```python
from build123d import *

# Parameters (mm, degrees)
CROQUIS1_W              = 50.8
CROQUIS1_H              = 6.31
SALIENTE_EXTRUIR1_DEPTH = 330.7
CROQUIS3_W              = 50.8
CROQUIS3_H              = 6.31
SALIENTE_EXTRUIR2_DEPTH = 644.51
CROQUIS4_W              = 50.8
CROQUIS4_H              = 6.31
CROQUIS8_R              = 6.5
CORTAR_EXTRUIR2_DEPTH   = 10
CROQUIS10_R             = 5
CORTAR_EXTRUIR4_DEPTH   = 50
CROQUIS11_R             = 5
CORTAR_EXTRUIR5_DEPTH   = 10


with BuildPart() as part:
    # Croquis1 → Saliente-Extruir1 (new body)
    with BuildSketch(Plane.XY):
        Rectangle(CROQUIS1_W, CROQUIS1_H)
    extrude(amount=SALIENTE_EXTRUIR1_DEPTH)

    # Croquis3 → Saliente-Extruir2 (add)
    with BuildSketch(Plane.XZ.offset(3.155)):
        with Locations((0, 3.155)):
            Rectangle(CROQUIS3_W, CROQUIS3_H)
    extrude(amount=-SALIENTE_EXTRUIR2_DEPTH)

    # Barrer1: sweep along a curve in space
    with BuildLine() as barrer1_path:
        Line((0, 641.355, 3.155), (0, 651.355, 3.155))
        Line((0, 651.355, 3.155), (0, 651.355, 95.765))
        Line((0, 651.355, 95.765), (0, 734.515, 95.765))
    # Croquis4 → Barrer1 (sweep)
    with BuildSketch(Plane(origin=(0, 641.355, 0), x_dir=(1, 0, 0), z_dir=(0, 1, 0))):
        with Locations((0, -3.155)):
            Rectangle(CROQUIS4_W, CROQUIS4_H)
    sweep(path=barrer1_path.line, transition=Transition.RIGHT)

    # Croquis8 → Cortar-Extruir2 (cut)
    with BuildSketch(Plane.XZ.offset(3.155)):
        with Locations(Location((0, 314.2, 0), (0, 0, 270))):
            Circle(CROQUIS8_R)
        with Locations(Location((0, 283.2, 0), (0, 0, 270))):
            Circle(CROQUIS8_R)
    extrude(amount=-CORTAR_EXTRUIR2_DEPTH, mode=Mode.SUBTRACT)

    # Croquis10 → Cortar-Extruir4 (cut)
    with BuildSketch(Plane.XY.offset(98.92)):
        with Locations((0, 700.515)):
            Circle(CROQUIS10_R)
    extrude(amount=-CORTAR_EXTRUIR4_DEPTH, mode=Mode.SUBTRACT)

    # Croquis11 → Cortar-Extruir5 (cut)
    with BuildSketch(Plane.XZ.offset(3.155)):
        with Locations(Location((0, 86.51, 0), (0, 0, 270))):
            Circle(CROQUIS11_R)
    extrude(amount=-CORTAR_EXTRUIR5_DEPTH, mode=Mode.SUBTRACT)


solid = part.part
```
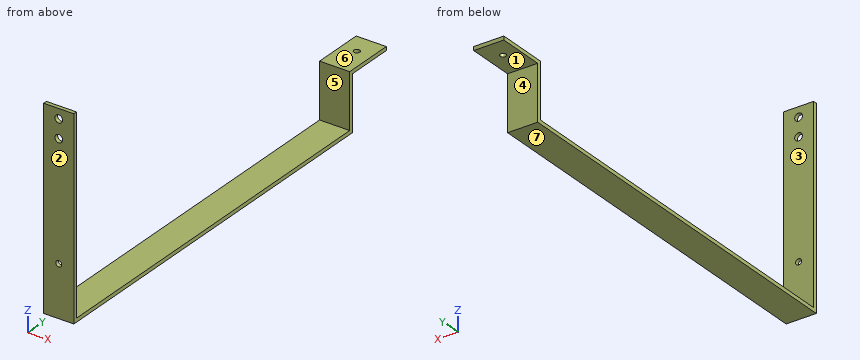
CAD build for the part. Positions are in the model's coordinates, mm. Face numbers are marked on the shaded views. A direction names the side the tool comes from. Round coordinates to 2 decimals unless told otherwise and drop trailing zeros. Loops run counter-clockwise (first coordinate to the right, second up) from the corner with the lowest first, then second, coordinate; pieces in that order, holes last. Notation, with made-up numbers: M 46,4.5 L 81,4.5 A14 cw 81,20.5 Z; hole C 17,39.5 d1. An arc over 180 degrees is marked long. Return JSON: item names as keys, results as strings. Group by question number.
(1) Saw through at B-B, the plane z = 66. List the corners of the cut face in (x, y) (3 decimals), and give its area (3 significant figures).
(2) Tool access for the marked faces 5, 6 and 7: list every direction of +Z, -Z, +X, -X, +Y, -Y with a clear straight run to the whole face (end or side of a thin tool).
(3) Saw through at A-A, the plane z = 283.2. List the corners of the cut face in (x, y) (3 decimals).
(4) Wall check: probe 1 along X at (y, z) = (1.5, 314.2); probe 2 along Y at (x, z) = (-20.5, 20) (3 decimals); probe 3 along X at (y, z) = (0.25, 86.51). Give the ranges that are in metal, low to high. Write a range as [from, to].
(5) Mould opens along Y. For the marked faces 1, 2, 3 and 4 say: +Y half, -Y half, draft (parallel to the pull), parting line (faces both ways), or undercut.
(6) Drop flat-ended pins along their axis: P1, Ø4, axis at x = -20, z = 270.5, coming from the +Y side (3 decimals); P2, Ø1.5, axis at x = -18.5, y = 389, coming from the +Z side; P3, Ø8, axis at x = -13.5, y = 401, coming from the -Z side; P4, Ø11.5, axis at x = 0, y = 700.515, coming from the +Z side. Give the stop position or say it passes through.
(7) Saw through at C-C, the plane z = 247. List the corners of the cut face in (x, y) (3 decimals), and give its area (3 significant figures).
(8) Saw through at D-D, the plane y = 486. List the corners of the cut face in (x, z), and give its area (3 significant figures).
Answer list:
{
 "1": {"outline": "M -25.4,-3.155 L 25.4,-3.155 L 25.4,3.155 L -25.4,3.155 Z; M -25.4,648.2 L 25.4,648.2 L 25.4,654.51 L -25.4,654.51 Z", "area": "641 mm2"},
 "2": {"face 5": "+Z, +X, -X", "face 6": "+Z, +X, -X, +Y", "face 7": "-Z, +X, -X, +Y, -Y"},
 "3": {"outline": "M -25.4,-3.155 L -6.5,-3.155 L -6.5,3.155 L -25.4,3.155 Z; M 6.5,-3.155 L 25.4,-3.155 L 25.4,3.155 L 6.5,3.155 Z"},
 "4": {"probe 1": "[-25.4, -6.5], [6.5, 25.4]", "probe 2": "[-3.155, 3.155], [648.2, 654.51]", "probe 3": "[-25.4, -5], [5, 25.4]"},
 "5": {"face 1": "draft", "face 2": "-Y half", "face 3": "undercut", "face 4": "+Y half"},
 "6": {"P1": "y = 3.155", "P2": "z = 6.31", "P3": "z = 0", "P4": "z = 98.92"},
 "7": {"outline": "M -25.4,-3.155 L 25.4,-3.155 L 25.4,3.155 L -25.4,3.155 Z", "area": "321 mm2"},
 "8": {"outline": "M -25.4,0 L 25.4,0 L 25.4,6.31 L -25.4,6.31 Z", "area": "321 mm2"}
}
